CAD build for the part. Positions are in the model's coordinates, mm. Face numbers are marked on the shaded views. Round coordinates to 2 decimals unless told otherwise and drop trailing zeros. Loops run counter-clockwise (first coordinate to the right, second up) from the corner with the lowest first, then second, coordinate; pieces in that order, holes last. Notation, with made-up numbers: M 34.5,-1 L 81.5,-1 A22 cw 81.5,34 Z; hole C 35,-25.5 d1. An arc over 180 degrees is marked long. One line per item, written item: value. Start each with the question number.
from build123d import *

# Parameters (mm, degrees)
F1_DEPTH = 9.525
F2_R     = 10.795
F3_DEPTH = 25.4


with BuildPart() as f1:
    # F0 (on Right) → F1 (new body, symmetric)
    with BuildSketch(Plane.YZ):
        with BuildLine():
            Line((-23.8125, 25.4), (-23.8125, -31.75))
            Line((-23.8125, -31.75), (23.8125, -31.75))
            Line((23.8125, -31.75), (23.8125, 25.4))
            ThreePointArc((23.8125, 25.4), (21.952628, 29.890128), (17.4625, 31.75))
            Line((17.4625, 31.75), (-17.4625, 31.75))
            ThreePointArc((-17.4625, 31.75), (-21.952628, 29.890128), (-23.8125, 25.4))
        make_face()
    extrude(amount=F1_DEPTH, both=True)

    # F2 (on face) → F3 (cut)
    with BuildSketch(Plane.YZ.offset(9.525)):
        with Locations((0, -3.175)):
            Circle(F2_R)
    extrude(amount=-F3_DEPTH, mode=Mode.SUBTRACT)


solid = f1.part
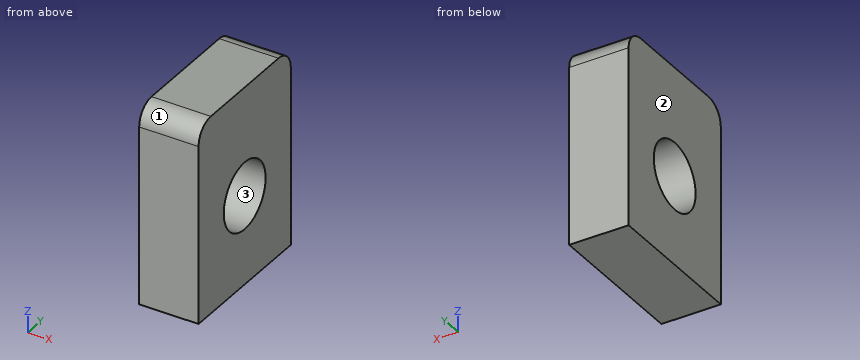
(1) Slice it at A-A, the plane y = 0. List the corners of the cut face in (x, z) (3 decimals), and give its area (3 significant figures).
(2) Slice it at C-C, the plane z = 1. List the corners of the cut face in (x, y) (1 decimal).
(3) Probe L1, parallel to Z at x = 0.5, y = 0; L2, parallel to Y at x = -2, z = -3.5; L3, parallel to Y at x = -3.5, z = 4. List the from-to ranges inside material, lowest first.
(4) Flat gauge pin, fed straight in: P1, Ø10, axis at y = 5, z = -5.5, coming from the -X side. Where does the tip first touch, or does it go through?
(5) Mould opens along Z. For the marked faces 1, 2 and 3 say: pulls with the +Z half, pulls with the -Z half, needs draft (parallel to the pull), parting line crosses it, or undercut.
Check result:
1. outline: M -9.525,-31.75 L 9.525,-31.75 L 9.525,-13.97 L -9.525,-13.97 Z; M -9.525,7.62 L 9.525,7.62 L 9.525,31.75 L -9.525,31.75 Z
1. area: 798 mm^2
2. outline: M -9.5,-23.8 L 9.5,-23.8 L 9.5,-10 L -9.5,-10 Z; M -9.5,10 L 9.5,10 L 9.5,23.8 L -9.5,23.8 Z
3. L1: z = -31.75 to -13.97, 7.62 to 31.75
3. L2: y = -23.81 to -10.79, 10.79 to 23.81
3. L3: y = -23.81 to -8.07, 8.07 to 23.81
4. P1: passes through
5. face 1: pulls with the +Z half
5. face 2: needs draft
5. face 3: undercut
